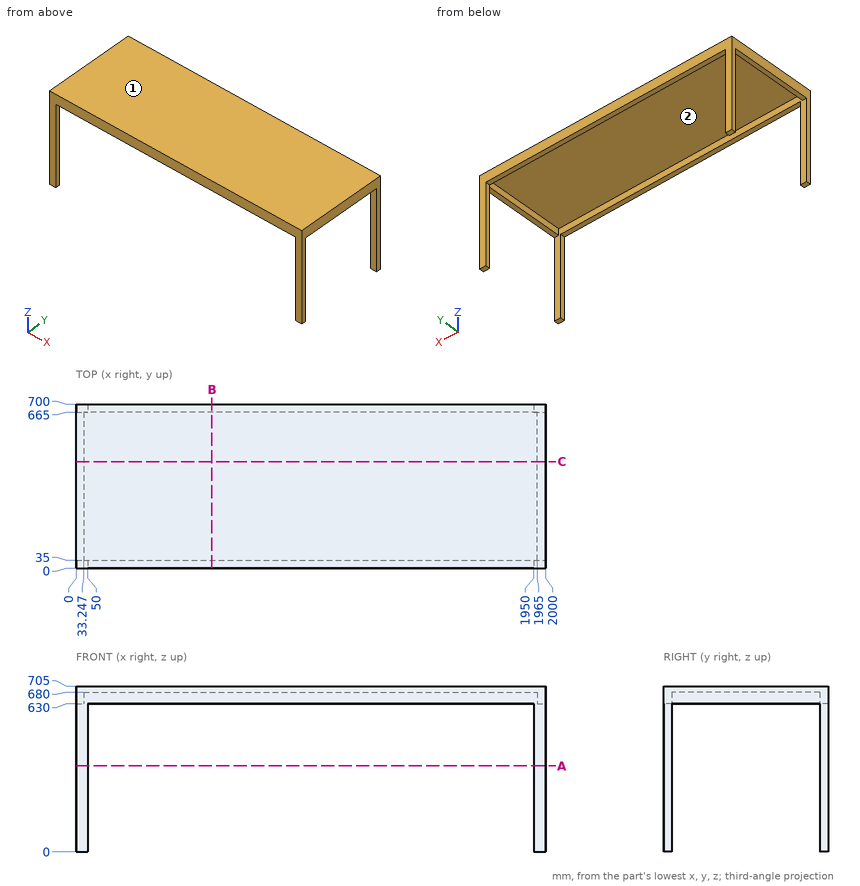
Job drawing, mm, ordinate dimensions from the low corner. One solid piece. Coordinates: 2 decimals unless noted, no trailing zeros. Order: outer loops, then holes, each group sorted by start corner. A loop starts at its lowest first (then second) coordinate and runs counter-clockwise, first axis right, second up. Notation, with made-up numbers: (3, -34.75) -> (44, -34.75) arc R25 cw to (44, 1.25) -> close; hole circle Ø8 at (-19, 82.25). An arc over 180 degrees is marked (long way). Put each result on its own line as item: value. Start each with the question number.
(1) Probe line 1 along X through (y, z) = (411.5, 655); line 2 along Z through (x, y) = (1706, 557). List the from-to ranges inside material, lowest first. Write a range as [from, to].
(2) Mould opens along X. For the marked faces 1 and 2 say: pulls with the +X half, pulls with the -X half, needs draft (parallel to the pull), parting line crosses it, or undercut.
(3) Pin check, flat tips, straight feed: pin 1 Ø17.5 at (x, y) = (758, 691) entering from -Z; pin 2 Ø4 at (x, y) = (571.5, 520.5) entering from -Z. Stop position of each tip, or through.
(4) Band-saw the part on C-C (y = 454.5). Give the cut face in (x, z), then the cut area to 3 significant figures.
(5) Band-saw the part on B-B (x = 578.5). Give the cut face in (y, z).
(6) Band-saw the part on A-A (z = 366.5). Give the cut face in (x, y), then the cut area to 3 significant figures.
Determined:
1. line 1: x = [0, 33.25], [1965, 2000]
1. line 2: z = [680, 705]
2. face 1: needs draft
2. face 2: undercut
3. pin 1: stops at z = 630
3. pin 2: stops at z = 680
4. outline: (0, 630) -> (33.25, 630) -> (33.25, 680) -> (1965, 680) -> (1965, 630) -> (2000, 630) -> (2000, 705) -> (0, 705) -> close
4. area: 53,400 mm²
5. outline: (0, 630) -> (35, 630) -> (35, 680) -> (665, 680) -> (665, 630) -> (700, 630) -> (700, 705) -> (0, 705) -> close
6. outline: (0, 0) -> (50, 0) -> (50, 35) -> (0, 35) -> close; (0, 665) -> (50, 665) -> (50, 700) -> (0, 700) -> close; (1950, 0) -> (2000, 0) -> (2000, 35) -> (1950, 35) -> close; (1950, 665) -> (2000, 665) -> (2000, 700) -> (1950, 700) -> close
6. area: 7,000 mm²
